Source: three-view drawing plus pictorial views. Frame: mm from the lowest corner of the part. Coordinates: 2 decimals unless noted, no trailing zeros. Order: outer loops, then holes, each group sorted by start corner. A loop starts at its lowest first (then second) coordinate and runs counter-clockwise, first axis right, second up. Notation, with made-up numbers: M 47.25,41 L 86.25,41 A22 cw 86.25,58 Z; hole C -22,-21 d4. An arc over 180 degrees is marked long. One line per question, with ' | ' between items.
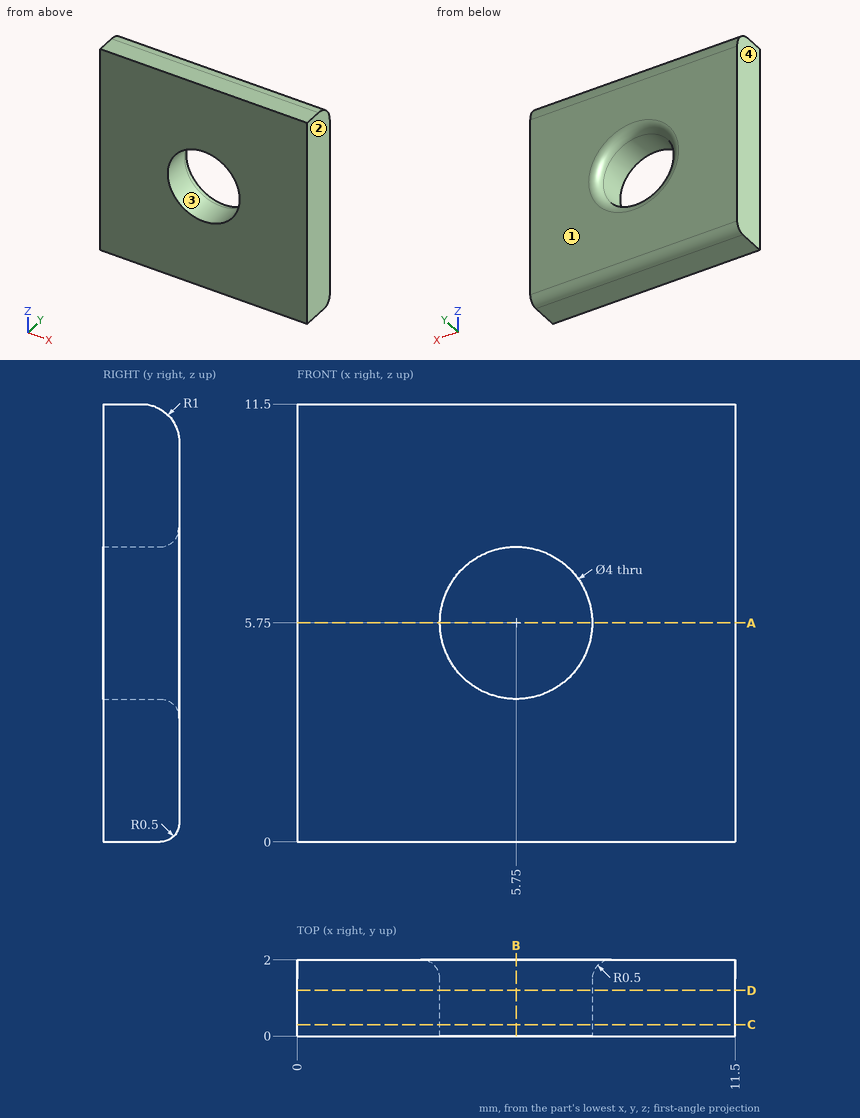
1. Section B-B, the plane x = 5.75. Output: boundary loops of the cut face in (y, z).
Response values:
outline: M 0,0 L 1.5,0 A0.5 ccw 2,0.5 L 2,3.25 A0.5 ccw 1.5,3.75 L 0,3.75 Z; M 0,7.75 L 1.5,7.75 A0.5 ccw 2,8.25 L 2,10.5 A1 ccw 1,11.5 L 0,11.5 Z
2. Draft query along X for the marked faces 1, 2, 3 and 4. Return one class per face: pulls with the +X half, pulls with the -X half, needs draft (parallel to the pull), parting line crosses it, or undercut.
Response values:
face 1: needs draft | face 2: pulls with the +X half | face 3: undercut | face 4: pulls with the -X half
3. Section C-C, the plane y = 0.3. Output: boundary loops of the cut face in (x, z), and give its area (3 significant figures).
Response values:
outline: M 0,0 L 11.5,0 L 11.5,11.5 L 0,11.5 Z; hole C 5.75,5.75 d4 | area: 120 mm^2
4. Section A-A, the plane z = 5.75. Output: boundary loops of the cut face in (x, y).
Response values:
outline: M 0,0 L 3.75,0 L 3.75,1.5 A0.5 ccw 3.25,2 L 0,2 Z; M 7.75,0 L 11.5,0 L 11.5,2 L 8.25,2 A0.5 ccw 7.75,1.5 Z
5. Pin query (flat end, axial travel): P1, Ø3.5, axis at x = 5.75, z = 5.75, coming from the +Y side. Return the tip coordinate at first contact, or that it passes through.
Response values:
P1: passes through
6. Material intervals for line 1 (X direction, y = 0.5, z = 5.75); line 2 (X direction, y = 0.65, z = 4.5), sorted ascending. Write a range as [from, to].
Response values:
line 1: x = [0, 3.75], [7.75, 11.5] | line 2: x = [0, 4.19], [7.31, 11.5]
7. Section D-D, the plane y = 1.2. Output: boundary loops of the cut face in (x, z), and give its area (3 significant figures).
Response values:
outline: M 0,0 L 11.5,0 L 11.5,11.48 L 0,11.48 Z; hole C 5.75,5.75 d4 | area: 119 mm^2
